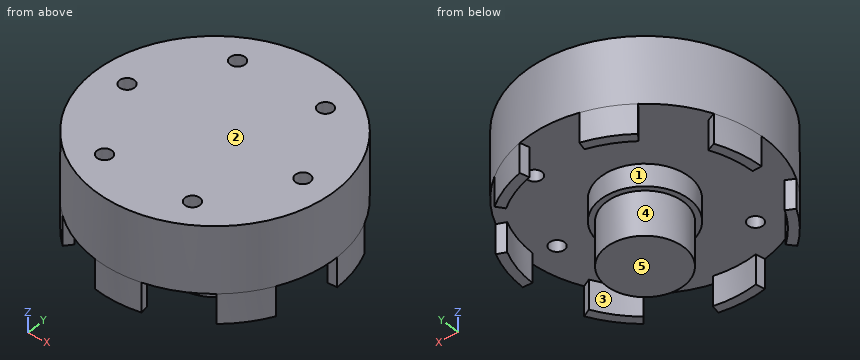
```python
from build123d import *

# Parameters (mm, degrees)
SKETCH1_R           = 10.5
BOSS_EXTRUDE1_DEPTH = 12
SKETCH2_R           = 12
BOSS_EXTRUDE2_DEPTH = 6
SKETCH3_R           = 32.5
BOSS_EXTRUDE3_DEPTH = 18
SKETCH4_R           = 2.025
CUT_EXTRUDE1_DEPTH  = 59.38236035
BOSS_EXTRUDE4_START = 8
BOSS_EXTRUDE4_DEPTH = 8


with BuildPart() as part:
    # Sketch1 → Boss-Extrude1 (new body)
    with BuildSketch(Plane.XY):
        Circle(SKETCH1_R)
    extrude(amount=BOSS_EXTRUDE1_DEPTH)

    # Sketch2 → Boss-Extrude2 (add)
    with BuildSketch(Plane.XY.offset(12)):
        Circle(SKETCH2_R)
    extrude(amount=BOSS_EXTRUDE2_DEPTH)

    # Sketch3 → Boss-Extrude3 (add)
    with BuildSketch(Plane.XY.offset(18)):
        Circle(SKETCH3_R)
    extrude(amount=BOSS_EXTRUDE3_DEPTH)

    # Sketch4 → Cut-Extrude1 (cut, through all)
    with BuildSketch(Plane.XY.offset(36)):
        with Locations((24.5, 0)):
            Circle(SKETCH4_R)
        with Locations((12.25, -21.217622393)):
            Circle(SKETCH4_R)
        with Locations((-12.25, -21.217622393)):
            Circle(SKETCH4_R)
        with Locations((-24.5, 0)):
            Circle(SKETCH4_R)
        with Locations((-12.25, 21.217622393)):
            Circle(SKETCH4_R)
        with Locations((12.25, 21.217622393)):
            Circle(SKETCH4_R)
    extrude(amount=-CUT_EXTRUDE1_DEPTH, mode=Mode.SUBTRACT)

    # Sketch5 → Boss-Extrude4 (add)
    with BuildSketch(Plane(origin=(0, 0, 18), x_dir=(-1, 0, 0), z_dir=(0, 0, -1)).offset(BOSS_EXTRUDE4_START)):
        with BuildLine():
            Line((27.716385975, 11.480502971), (30.026084807, 12.437211552))
            ThreePointArc((30.026084807, 12.437211552), (31.875521613, 6.340435466), (32.5, 0))
            Line((32.5, 0), (30, 0))
            ThreePointArc((30, 0), (29.423558412, 5.85270966), (27.716385975, 11.480502971))
        make_face()
        with BuildLine():
            Line((26.256702657, -14.511566613), (28.444761212, -15.720863831))
            ThreePointArc((28.444761212, -15.720863831), (24.831214714, -20.968089465), (20.26341856, -25.40952318))
            Line((20.26341856, -25.40952318), (18.704694056, -23.454944474))
            ThreePointArc((18.704694056, -23.454944474), (22.921121275, -19.355159506), (26.256702657, -14.511566613))
        make_face()
        with BuildLine():
            Line((5.025186699, -29.576130556), (5.443952257, -32.040808102))
            ThreePointArc((5.443952257, -32.040808102), (-0.911503329, -32.487215357), (-7.231930354, -31.685157146))
            Line((-7.231930354, -31.685157146), (-6.675628019, -29.247837365))
            ThreePointArc((-6.675628019, -29.247837365), (-0.841387688, -29.988198791), (5.025186699, -29.576130556))
        make_face()
        with BuildLine():
            Line((-19.990397339, -22.369264946), (-21.656263783, -24.233370359))
            ThreePointArc((-21.656263783, -24.233370359), (-25.967840774, -19.542805467), (-29.281488207, -14.101221521))
            Line((-29.281488207, -14.101221521), (-27.029066037, -13.016512174))
            ThreePointArc((-27.029066037, -13.016512174), (-23.970314561, -18.039512739), (-19.990397339, -22.369264946))
        make_face()
        with BuildLine():
            Line((-29.952804451, 1.682113417), (-32.448871488, 1.822289535))
            ThreePointArc((-32.448871488, 1.822289535), (-31.469864469, 8.11773554), (-29.281488207, 14.101221521))
            Line((-29.281488207, 14.101221521), (-27.029066037, 13.016512174))
            ThreePointArc((-27.029066037, 13.016512174), (-29.049105664, 7.493294345), (-29.952804451, 1.682113417))
        make_face()
        with BuildLine():
            Line((-17.360138885, 24.466826069), (-18.806817126, 26.505728241))
            ThreePointArc((-18.806817126, 26.505728241), (-13.27443835, 29.665456114), (-7.231930354, 31.685157146))
            Line((-7.231930354, 31.685157146), (-6.675628019, 29.247837365))
            ThreePointArc((-6.675628019, 29.247837365), (-12.253327708, 27.383497952), (-17.360138885, 24.466826069))
        make_face()
        with BuildLine():
            Line((8.305065343, 28.827519658), (8.997154121, 31.229812963))
            ThreePointArc((8.997154121, 31.229812963), (14.916910595, 28.874483169), (20.26341856, 25.40952318))
            Line((20.26341856, 25.40952318), (18.704694056, 23.454944474))
            ThreePointArc((18.704694056, 23.454944474), (13.769455934, 26.653369079), (8.305065343, 28.827519658))
        make_face()
    extrude(amount=-BOSS_EXTRUDE4_DEPTH)


solid = part.part
```
Input: part model. Units: mm. Frame: model coordinates. Face numbers are marked on the shaded views. A direction names the side the tool comes from. Give positions to 0.01 mm unless a question says otherwise; leave off trailing zeros. Order: outer loops, then holes, each group sorted by start corner. A loop starts at its lowest first (then second) coordinate and runs counter-clockwise, first axis right, second up.
1. Draft query along Y for the marked faces 1, 2 and 3. Return one class per face: released by +Y, released by -Y, zero draft, split by the parting line, or undercut.
Computed:
face 1: undercut
face 2: zero draft
face 3: released by +Y
2. Cut plane C-C (x = -24.5). Return loops of the section in (y, z) (3 decimals), and give its area (3 significant figures).
Computed:
outline: (-21.354, 10) - (-17.313, 10) - (-17.313, 18) - (-2.025, 18) - (-2.025, 36) - (-21.354, 36) - close; (2.025, 18) - (21.354, 18) - (21.354, 36) - (2.025, 36) - close
area: 728 mm2
3. Pin query (flat end, axial travel): pin 1 Ø1.6 at (x, y) = (3.5, -30.5) entering from -Z; pin 2 Ø10 at (y, z) = (-19.5, 18) entering from +X; pin 3 Ø4 at (x, z) = (3, 32) entering from -Y. Return the tip coordinate at first contact, or that it passes through.
Computed:
pin 1: stops at z = 10
pin 2: stops at x = 29.09
pin 3: stops at y = -32.48
4. Set-up query: the marked faces 4 and 5. Return all of +Z, -Z, +X, -X, +Y, -Y with unobstructed straight access to the full face (end or side cutting, diameter ignored); none if empty.
Computed:
face 4: -Z
face 5: -Z, +X, -X, +Y, -Y
5. Cut plane A-A (z = 11). State how many separate pieces and enclosed holes the cut face has, and give its area (3 significant figures).
Computed:
separate pieces: 8
enclosed holes: 0
area: 561 mm2
6. Line query: probe 1 along Y at (x, z) = (12.25, 27.5); probe 2 along Y at (x, z) = (14, 34.5); probe 3 along Y at (x, z) = (-0.5, 17). Output: solid intervals per line, ascending.
Computed:
probe 1: y = -30.1 to -23.24, -19.19 to 19.19, 23.24 to 30.1
probe 2: y = -29.33 to -22.24, -20.2 to 20.2, 22.24 to 29.33
probe 3: y = -32.5 to -30, -11.99 to 11.99
7. Cut plane B-B (y = -20). Return loops of the section in (x, z), and give its area (3 significant figures).
Computed:
outline: (-25.62, 10) - (-22.36, 10) - (-22.36, 18) - (-13.87, 18) - (-13.87, 36) - (-25.62, 36) - close; (-10.63, 18) - (10.63, 18) - (10.63, 36) - (-10.63, 36) - close; (13.87, 18) - (22.36, 18) - (22.36, 10) - (25.62, 10) - (25.62, 36) - (13.87, 36) - close
area: 858 mm2
